Input: part model. Units: mm. Frame: model coordinates. Round coordinates to 2 decimals unless told otherwise and drop trailing zeros. Loops run counter-clockwise (first coordinate to the right, second up) from the corner with the lowest first, then second, coordinate; pieces in that order, holes last.
(1) Cut plane A-A, the plane y = 1.9. Output: boundary loops of the cut face in (x, z), and give its area (3 significant figures).
(2) Cut plane B-B, the plane x = 1.25. Output: boundary loops of the cut face in (y, z), and give its area (3 significant figures).
(3) First-contact query: pin 1 Ø1 at (x, y) = (-1.5, 1) entering from -Z. Flat tip, straight axial feed; report the tip coordinate or a pass-through.
(4) Line query: line 1 (X direction, y = 1.45, z = -6.5); line 2 (X direction, y = 3.3, z = 0); line 3 (Z direction, x = 0.75, y = 3.4). Output: solid intervals per line, ascending.
(5) Cut plane C-C, the plane z = -0.75. Output: boundary loops of the cut face in (x, y), and give its area (3 significant figures).
Autodesk Fusion 360 part; units mm, degrees
sketch "Skizze1" plane through (0, 0, 0) normal (0, 1, 0) x (1, 0, 0)
  line L0 (0, 7.7) -> (0, 0)
  line L1 (0, 7.7) -> (0.0094, 3.85)
  line L2 (0, 7.7) -> (0, 0)
  line L3 (-0.0094, -0.25) -> (3.5413, 1.8)
  line L4 (3.5413, 1.8) -> (3.5413, 5.9)
  line L5 (3.5413, 5.9) -> (-0.0095, 7.95)
  line L6 (-0.0095, 7.95) -> (-3.5602, 5.9)
  line L7 (-3.5602, 5.9) -> (-3.5602, 1.8)
  line L8 (-3.5602, 1.8) -> (-0.0094, -0.25)
  point P0 (0.0094, 3.85)
  point P1 (-0.0094, 3.85)
  dimension "d1" = 7.7
  dimension "d3" = 3.85
  dimension "d4" = 7.7
  dimension "d5" = 4.1
  dimension "d6" = 4.1
  dimension "d7" = 4.1
  dimension "d8" = 4.1
  dimension "d9" = 4.1
  dimension "d10" = 4.1
extrude "Extrusion1" add sketch "Skizze1" along normal blind 4 makes body 1
copy_body "Körper->Berechn1" bodies 1 removing the originals makes body 2 in component "Component"
component "Component" placed x (1, 0, 0) y (0, 1, 0) z (0, 0, 1) at (0, 0, 0)
Reported:
1. outline: (-3.56, -5.9) - (-0.01, -7.95) - (3.54, -5.9) - (3.54, -1.8) - (-0.01, 0.25) - (-3.56, -1.8) - close
1. area: 43.7 mm2
2. outline: (0, -7.22) - (4, -7.22) - (4, -0.48) - (0, -0.48) - close
2. area: 27.0 mm2
3. pin 1: stops at z = -7.38
4. line 1: x = -2.52 to 2.5
4. line 2: x = -0.44 to 0.42
4. line 3: z = -7.51 to -0.19
5. outline: (-1.74, 0) - (1.72, 0) - (1.72, 4) - (-1.74, 4) - close
5. area: 13.9 mm2
